Autodesk Inventor part; units mm, degrees
ref_plane "YZ Plane" through (0, 0, 0) normal (1, 0, 0) x (0, 1, 0)
ref_plane "XZ Plane" through (0, 0, 0) normal (0, 1, 0) x (-1, 0, 0)
ref_plane "XY Plane" through (0, 0, 0) normal (0, 0, 1) x (1, 0, 0)
sketch "Sketch1" plane through (0, 0, 0) normal (0, 1, 0) x (-1, 0, 0)
  circle A0 centre (0, 0) radius 8.125
  circle A1 centre (0, 0) radius 6.625
  dimension "d0" = 16.25
  dimension "d1" = 13.25
sketch "Sketch3" plane through (0, 0, 0) normal (0, 0, 1) x (1, 0, 0)
  line L0 (8.125, 0) -> (8.125, 20)
  line L1 (8.125, 0) -> (28.125, 0) construction
  arc A0 (8.125, 20) -> (-11.875, 40) centre (-11.875, 20) ccw
  line L2 (-11.875, 40) -> (-31.875, 40)
  point P0 (0, 0)
  dimension "d5" = 20
  dimension "d6" = 90
  dimension "d7" = 20
  dimension "d10" = 20
sweep "Sweep1" add profiles "Sketch1" path "Sketch3"
properties part number "Effector Wire Conduit"
Design review of the part built by this model. Coordinates are the model's own, in mm. A direction names the side the tool comes from. Round coordinates to 2 decimals unless told otherwise and drop trailing zeros. Write each loop counter-clockwise with the first axis right and the second up, starting at its lowest first coordinate (ties: lowest second). Pieces come first, ordered by that corner, then holes.
Item 1: Consider section B-B on x = -17. Give the boundary of the cut face in (y, z) (3 decimals), and give its area (3 significant figures).
Item 2: Consider section A-A on z = 0. Give the boundary of the cut face in (x, y) (3 decimals), and give its area (3 significant figures).
Item 3: For pin 1 Ø2 at (x, z) = (4, 1) entering from +Y; pin 2 Ø8 at (y, z) = (5.5, 5) entering from +X; pin 3 Ø3 at (y, z) = (17.5, 6) entering from +X (3 decimals), all flat-tipped, find the tip position at first contact; note any pin that passes through.
Item 4: Wall thickness on L1, parallel to Z at x = 0, y = 4 (3 decimals); L2, parallel to X at y = 24.5, z = 5.5; L3, parallel to X at y = 2, z = -3.5 (1 decimal): over which ranges is each line inside the solid? List them lowest first.
Item 5: For faces 1 (the cylindrical face through (-22.015, 38.494, 0.291)), 2 (the flat face through (0, 0, -7)), list the 3-axis set-ups (+Z, -Z, +X, -X, +Y, -Y) from which the entire face can be reached by the end or side of a thin tool; tool diameter is ignored.
Item 6: Consider section C-C on y = 4. Give the boundary of the cut face in (x, z) (3 decimals).
Item 7: Draft analysis for pull direction X (two halves, no side actions). For faces 3 (the cylindrical face through (-3.562, 10.14, 5.586)), 4 (the flat face through (-31.875, 32, 7)), 5 (the cylindrical face through (-7.75, 10.14, 2.44)), state which applies: released by +X, released by -X, zero draft, split by the parting line, or undercut.
Check values:
1. outline: circle Ø16.25 at (31.875, 0); hole circle Ø13.25 at (31.875, 0)
1. area: 69.5 mm2
2. outline: (-31.875, 23.75) - (-11.875, 23.75) arc R3.75 cw to (-8.125, 20) - (-8.125, 0) - (-6.625, 0) - (-6.625, 20) arc R5.25 ccw to (-11.875, 25.25) - (-31.875, 25.25) - close; (-31.875, 38.5) - (-11.875, 38.5) arc R18.5 cw to (6.625, 20) - (6.625, 0) - (8.125, 0) - (8.125, 20) arc R20 ccw to (-11.875, 40) - (-31.875, 40) - close
2. area: 176 mm2
3. pin 1: stops at y = 33.29
3. pin 2: stops at x = 8.06
3. pin 3: stops at x = 6.765
4. L1: z = -8.125 to -6.625, 6.625 to 8.125
4. L2: x = -8.07 to -5.04, 3.03 to 5.4
4. L3: x = -7.3 to -5.6, 5.6 to 7.3
5. face 1: -X
5. face 2: +Z, -Z, +X, -X, -Y
6. outline: circle Ø16.25 at (0, 0); hole circle Ø13.25 at (0, 0)
7. face 3: undercut
7. face 4: released by -X
7. face 5: split by the parting line
